```python
from build123d import *

# Parameters (mm, degrees)
F0_R     = 45.5
F0_R_2   = 38.75
F1_DEPTH = 5
F0_R_3   = 31
F2_DEPTH = 45


with BuildPart() as f1:
    # F0 (on Top) → F1 (new body)
    with BuildSketch(Plane.XY):
        Circle(F0_R)
        Circle(F0_R_2, mode=Mode.SUBTRACT)
    extrude(amount=F1_DEPTH)

    # F0 (on Top) → F2 (join)
    with BuildSketch(Plane.XY):
        Circle(F0_R_2)
        with Locations((-5.749998, 0.004193)):
            Circle(F0_R_3, mode=Mode.SUBTRACT)
        with BuildLine():
            ThreePointArc((33.258886, -11.5), (32.965992, -12.207107), (32.258886, -12.5))
            Line((32.258886, -12.5), (29.258886, -12.5))
            ThreePointArc((29.258886, -12.5), (28.551779, -12.207107), (28.258886, -11.5))
            Line((28.258886, -11.5), (28.258886, 11.5))
            ThreePointArc((28.258886, 11.5), (28.551779, 12.207107), (29.258886, 12.5))
            Line((29.258886, 12.5), (32.258886, 12.5))
            ThreePointArc((32.258886, 12.5), (32.965992, 12.207107), (33.258886, 11.5))
            Line((33.258886, 11.5), (33.258886, -11.5))
        make_face(mode=Mode.SUBTRACT)
    extrude(amount=F2_DEPTH)


solid = f1.part
```
Source: CAD feature listing. Evaluate the final solid. Frame: model axes, mm. A direction names the side the tool comes from. Give positions to 0.01 mm unless a question says otherwise; leave off trailing zeros. Write each loop counter-clockwise with the first axis right and the second up, starting at its lowest first coordinate (ties: lowest second). Pieces come first, ordered by that corner, then holes. Notation, with made-up numbers: (88.25, 72) - (112.25, 72) arc R33 ccw to (112.25, 100) - close; hole circle Ø5 at (59.25, 50). An arc over 180 degrees is marked (long way). One line per item, written item: value. Start each with the question number.
Q1. Section query A-A, the plane x = 11.5. Return the cut outline in (y, z).
Q2. Draft query along Y for faces 1 (the face through (20, -20, 0)), 2 (the face through (-8.4, -37.83, 24.72)), 3 (the face through (33.259, 0, 22)), 4 (the face through (31, -12.5, 22)). Return one class per face: +Y half, -Y half, draft (parallel to the pull), parting line (faces both ways), or undercut.
Q3. Section query B-B, the plane y = -9. Return the cut outline in (x, z).
Q4. First-contact query: pin 1 Ø8 at (y, z) = (-16, 12.5) entering from -X; pin 2 Ø1.5 at (x, z) = (-35, 4.5) entering from -Y; pin 3 Ø4 at (x, z) = (10, 23) entering from -Y; pin 4 Ø1 at (x, y) = (0.5, -28) entering from -Z (3 decimals). Flat tips, straight axial feed; report the tip coordinate or a pass-through.
Q5. Section query C-C, the plane y = -29.5. Return the cut outline in (x, z), then the cut area to 3 significant figures.
Q6. Section query D-D, the plane z = 12. Return the cut outline in (x, y), then the cut area to 3 significant figures.
Q7. Material intervals for probe 1 along X at (y, z) = (11, 41.5); probe 2 along X at (y, z) = (9.5, 42.5); probe 3 along Y at (x, z) = (-15, 37), sorted ascending. Write a range as from..to.
Q8. Set-up query: faces 5 (the face through (33.5, 20.4, 5)), 6 (the face through (26, 3, 45)), 7 (the face through (31, 12.5, 22)). Return all of +Z, -Z, +X, -X, +Y, -Y with unobstructed straight access to the full face (end or side cutting, diameter ignored); none if empty.
Answer:
1. outline: (-44.02, 0) - (-25.75, 0) - (-25.75, 45) - (-37, 45) - (-37, 5) - (-44.02, 5) - close; (25.76, 0) - (44.02, 0) - (44.02, 5) - (37, 5) - (37, 45) - (25.76, 45) - close
2. face 1: draft
2. face 2: parting line
2. face 3: undercut
2. face 4: undercut
3. outline: (-44.6, 0) - (-35.41, 0) - (-35.41, 45) - (-37.69, 45) - (-37.69, 5) - (-44.6, 5) - close; (23.91, 0) - (28.26, 0) - (28.26, 45) - (23.91, 45) - close; (33.26, 0) - (44.6, 0) - (44.6, 5) - (37.69, 5) - (37.69, 45) - (33.26, 45) - close
4. pin 1: stops at x = -36.85
4. pin 2: stops at y = -29.95
4. pin 3: stops at y = -37.92
4. pin 4: passes through
5. outline: (-34.64, 0) - (-15.26, 0) - (-15.26, 45) - (-25.13, 45) - (-25.13, 5) - (-34.64, 5) - close; (3.76, 0) - (34.64, 0) - (34.64, 5) - (25.13, 5) - (25.13, 45) - (3.76, 45) - close
5. area: 1,500 mm2
6. outline: circle Ø77.5 at (0, 0); hole circle Ø62 at (-5.75, 0); hole (28.26, -11.5) arc R1 ccw to (29.26, -12.5) - (32.26, -12.5) arc R1 ccw to (33.26, -11.5) - (33.26, 11.5) arc R1 ccw to (32.26, 12.5) - (29.26, 12.5) arc R1 ccw to (28.26, 11.5) - close
6. area: 1,570 mm2
7. probe 1: x = -37.16..-34.73, 23.23..28.26, 33.26..37.16
7. probe 2: x = -37.57..-35.26, 23.76..28.26, 33.26..37.57
7. probe 3: y = -35.73..-29.58, 29.59..35.73
8. face 5: +Z
8. face 6: +Z, +X, -X, +Y, -Y
8. face 7: +Z, -Z
